Verification items for the finished model (mm, model axes). Face numbers are marked on the shaded views. A direction names the side the tool comes from. Give positions to 0.01 mm unless a question says otherwise; leave off trailing zeros. Order: outer loops, then holes, each group sorted by start corner. A loop starts at its lowest first (then second) coordinate and runs counter-clockwise, first axis right, second up. Notation, with made-up numbers: (-20.75, 5.25) -> (28.25, 5.25) arc R13 cw to (28.25, 12.25) -> close; hole circle Ø11 at (11, 16). An arc over 180 degrees is marked (long way). Write each question's results on one line, items separated by ' | '. Start each with the question number.
1. Set-up check for the marked faces 1, 2, 3 and 4: record each of +Z, -Z, +X, -X, +Y, -Y from which the full face is reachable in a straight line by a thin tool's end or side.
2. Mould release check, pull along Y, two halves, no side actions. Record for the marked faces 5, 6 and 7: +Y half, -Y half, draft (parallel to the pull), parting line (faces both ways), or undercut.
3. Depth check by flat-ended pin: pin 1 Ø4 at (x, y) = (16, 34) entering from -Z; pin 2 Ø1 at (x, z) = (33.5, 21) entering from +Y; pin 3 Ø8 at (x, z) = (-37.5, -11) entering from -Y. Enter the tip coordinate at first touch or a pass-through.
4. Cross-section at A-A, the plane y = 0. Enter the section's corners in (x, z).
5. Cross-section at D-D, the plane y = -20. Enter the section's corners in (x, z), then the cut area to 3 significant figures.
6. Cross-section at C-C, the plane z = -9. Enter the section's corners in (x, y), then the cut area to 3 significant figures.
7. Material ranges on L1, parallel to X at y = 8, z = 0; L2, parallel to Z at x = 19.5, y = 39; L3, parallel to Z at x = -4, y = 0, recorded low to high. Write a range as from..to.
from build123d import *

# Parameters (mm, degrees)
SKETCH1_R           = 20
BOSS_EXTRUDE1_DEPTH = 15
BOSS_EXTRUDE2_DEPTH = 50
CUT_EXTRUDE1_DEPTH  = 210.975927192


with BuildPart() as part:
    # Sketch1 → Boss-Extrude1 (new, symmetric)
    with BuildSketch(Plane(origin=(0, 0, 0), x_dir=(1, 0, 0), z_dir=(0, 1, 0))):
        with BuildLine():
            ThreePointArc((50, 0), (0, 50), (-50, 0))
            Line((-50, 0), (-50, -60))
            Line((-50, -60), (50, -60))
            Line((50, -60), (50, 0))
        make_face()
        with Locations(Location((0, 0, 0), (0, 0, 270))):
            Circle(SKETCH1_R, mode=Mode.SUBTRACT)
    extrude(amount=BOSS_EXTRUDE1_DEPTH, both=True)

    # Sketch1_3 → Boss-Extrude2 (add, symmetric)
    with BuildSketch(Plane(origin=(0, 0, 0), x_dir=(1, 0, 0), z_dir=(0, 1, 0))):
        Polygon((0, -60), (-50, -60), (-50, -100), (-15, -100), (-15, -193.3), (0, -193.3), align=None)
        Polygon((50, -60), (0, -60), (0, -193.3), (15, -193.3), (15, -100), (50, -100), align=None)
    extrude(amount=BOSS_EXTRUDE2_DEPTH, both=True)

    # Sketch2 → Cut-Extrude1 (cut, through all)
    with BuildSketch(Plane(origin=(15, 0, 0), x_dir=(0, 0, -1), z_dir=(1, 0, 0))):
        with BuildLine():
            Line((-193.3, 50), (-193.3, 25.002199903))
            ThreePointArc((-193.3, 25.002199903), (-174.998900024, 43.301905242), (-150, 50))
            Line((-150, 50), (-193.3, 50))
        make_face()
        with BuildLine():
            ThreePointArc((-150, -25), (-125, 0), (-150, 25))
            Line((-150, 25), (-193.3, 25))
            Line((-193.3, 25), (-193.3, -25))
            Line((-193.3, -25), (-150, -25))
        make_face()
        with BuildLine():
            ThreePointArc((-150, -50), (-174.998900024, -43.301905242), (-193.3, -25.002199903))
            Line((-193.3, -25.002199903), (-193.3, -50))
            Line((-193.3, -50), (-150, -50))
        make_face()
    extrude(amount=-CUT_EXTRUDE1_DEPTH, mode=Mode.SUBTRACT)


solid = part.part
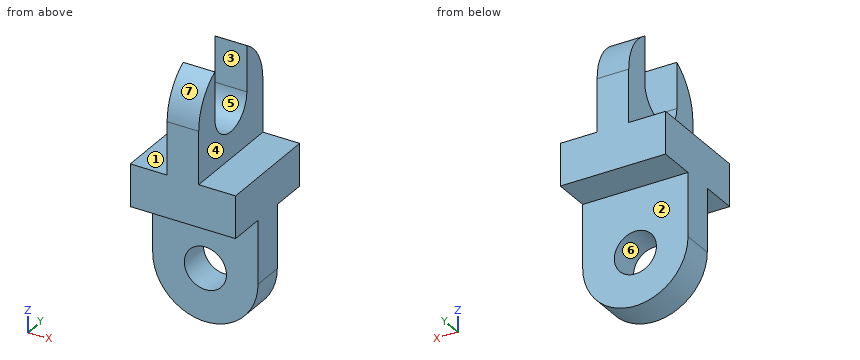
Results below:
1) face 1: +Z, -X, +Y, -Y | face 2: -Z, +X, -X, +Y | face 3: +Z, +X, -X | face 4: +Z, +X, +Y, -Y
2) face 5: undercut | face 6: draft | face 7: -Y half
3) pin 1: stops at z = 60 | pin 2: stops at y = 15 | pin 3: stops at y = -15
4) outline: (-50, 0) arc R50 ccw to (50, 0) -> (50, 100) -> (15, 100) -> (15, 125) -> (-15, 125) -> (-15, 100) -> (-50, 100) -> close; hole circle Ø40 at (0, 0)
5) outline: (-50, 60) -> (50, 60) -> (50, 100) -> (15, 100) -> (15, 135) -> (-15, 135) -> (-15, 100) -> (-50, 100) -> close | area: 5,050 mm²
6) outline: (-49.18, -15) -> (-17.86, -15) -> (-17.86, 15) -> (-49.18, 15) -> close; (17.86, -15) -> (49.18, -15) -> (49.18, 15) -> (17.86, 15) -> close | area: 1,880 mm²
7) L1: x = -50..-20, 20..50 | L2: z = 60..100 | L3: z = -49.84..-19.6, 19.6..125
